Geometry: see drawing. Coordinates: mm, zero at the bounding-box minimum. Coordinates: 2 decimals unless noted, no trailing zeros. Write each loop counter-clockwise with the first axis right and the second up, starting at its lowest first coordinate (ties: lowest second). Pieces come first, ordered by that corner, then holes. Notation, with made-up numbers: (-36.75, 41.5) - (-29.75, 41.5) arc R36 cw to (-29.75, 75.5) - close; hole circle Ø4 at (-23.75, 60). An arc over 180 degrees is marked (long way). One line per question, with ' | ' between items. Start each with the question number.
Q1. Cut plane B-B, the plane x = 43.5. Return loops of the section in (y, z), plus the area to 3 significant figures.
Q2. Line query: line 1 (Z direction, x = 28.5, y = 24); line 2 (Z direction, x = 31.5, y = 21) (1 decimal). Output: solid intervals per line, ascending.
Q3. Contact query for flat-ended pins moving along their axis: P1, Ø2, axis at x = 13.5, y = 19.5, coming from the +Z side; P2, Ø1, axis at x = 68.5, y = 10, coming from the +Z side (1 decimal). Output: stop coordinate, or through.
Q4. Cut plane A-A, the plane y = 23. Return loops of the section in (x, z) (1 decimal), plus the area to 3 significant figures.
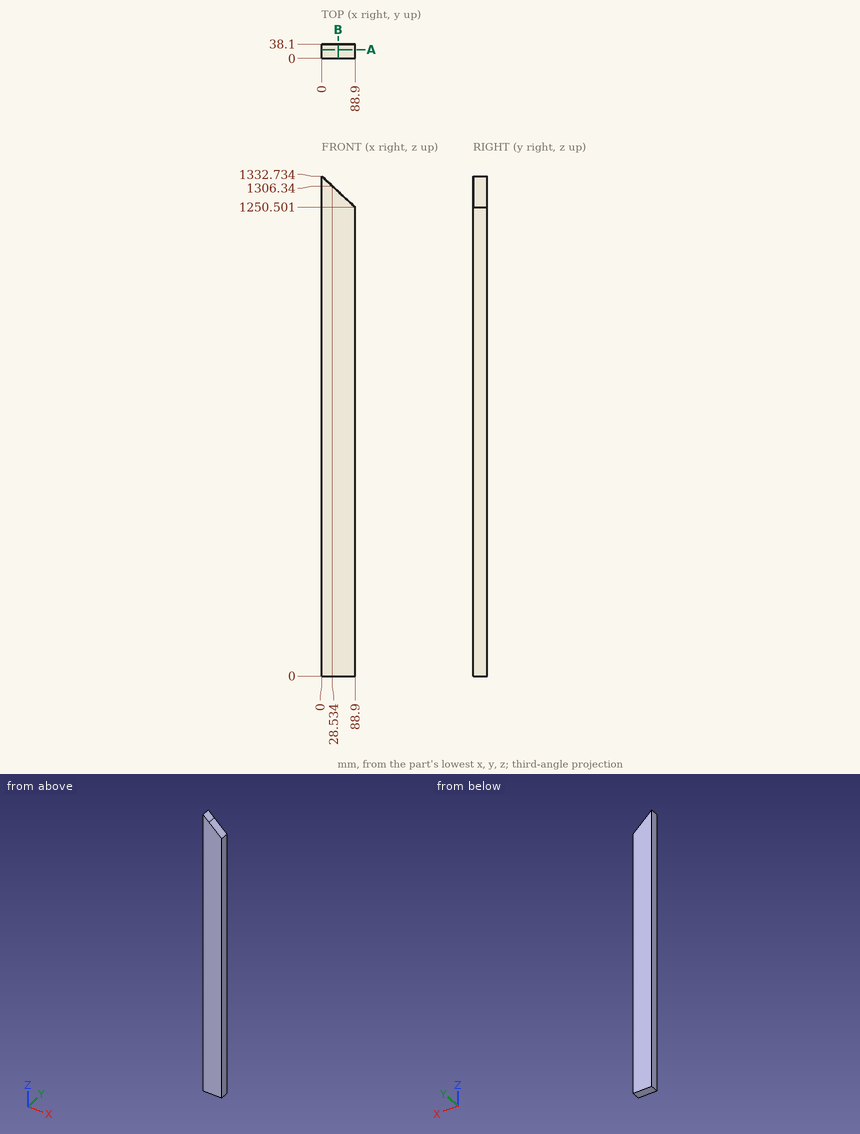
Reply:
1) outline: (0, 0) - (38.1, 0) - (38.1, 1292.5) - (0, 1292.5) - close | area: 49,200 mm^2
2) line 1: z = 0 to 1306.37 | line 2: z = 0 to 1303.6
3) P1: stops at z = 1321.17 | P2: stops at z = 1269.8
4) outline: (0, 0) - (88.9, 0) - (88.9, 1250.5) - (0, 1332.7) - close | area: 115,000 mm^2
